Source: CAD feature listing. Evaluate the final solid. Frame: model axes, mm. A direction names the side the tool comes from. Round coordinates to 2 decimals unless told otherwise and drop trailing zeros. Loops run counter-clockwise (first coordinate to the right, second up) from the corner with the lowest first, then second, coordinate; pieces in that order, holes last. Notation, with made-up numbers: (-16.5, 30) - (1.5, 30) arc R16 cw to (1.5, 39) - close; hole circle Ø10 at (-27.75, 7.5). An arc over 180 degrees is marked (long way). Use CSV: the item, a comma, the result in double quotes. Start each with the question number.
from build123d import *

# Parameters (mm, degrees)
F0_R     = 6.35
F0_R_2   = 4.7625
F1_DEPTH = 6.35
F2_R     = 32.0379747342
F3_ANGLE = 180


with BuildPart() as f1:
    # F0 (on Front) → F1 (new body)
    with BuildSketch(Plane.XZ):
        with BuildLine():
            add(Edge.make_bspline(
                [(-44.9317906939, -75.2959670142), (-42.504350489, -76.9309330496), (-40.0815580843, -78.574281615), (-37.0058182453, -78.848974732)],
                knots=[0, 0, 0, 0, 0.304878312, 0.304878312, 0.304878312, 0.304878312], degree=3))
            Line((-37.0058182453, -78.848974732), (-35.1899303496, -78.848974732))
            Line((-35.1899303496, -78.848974732), (138.0456507325, -78.848974732))
            ThreePointArc((138.0456507325, -78.848974732), (107.5329699783, -68.6644436224), (89.25483042, -42.1944988733))
            ThreePointArc((89.25483042, -42.1944988733), (72.9581507325, -28.048974732), (89.25483042, -13.9034505906))
            ThreePointArc((89.25483042, -13.9034505906), (107.5329699783, 12.5664941585), (138.0456507325, 22.751025268))
            Line((138.0456507325, 22.751025268), (-29.5108688384, 22.751025268))
            ThreePointArc((-29.5108688384, 22.751025268), (-23.7287326375, -9.9063657522), (-37.9096431739, -39.8870272468))
            ThreePointArc((-37.9096431739, -39.8870272468), (-36.8982172715, -41.4219866867), (-36.5434579184, -43.2256575657))
            ThreePointArc((-36.5434579184, -43.2256575657), (-39.6962005674, -47.7078542952), (-44.9802400795, -46.2556834486))
            ThreePointArc((-44.9802400795, -46.2556834486), (-45.2388732076, -46.4494635579), (-45.4986485664, -46.6417097247))
            ThreePointArc((-45.4986485664, -46.6417097247), (-44.8982077868, -47.9076096174), (-44.6921152233, -49.2934514277))
            ThreePointArc((-44.6921152233, -49.2934514277), (-48.2687720926, -53.9059542537), (-53.62657499, -51.5904403165))
            ThreePointArc((-53.62657499, -51.5904403165), (-53.9605685551, -51.7543648971), (-54.2956711641, -51.9160102225))
            ThreePointArc((-54.2956711641, -51.9160102225), (-54.0112987886, -52.8294235617), (-53.9152156835, -53.781242669))
            ThreePointArc((-53.9152156835, -53.781242669), (-57.9302793656, -58.484724911), (-63.2056073689, -55.2575905738))
            ThreePointArc((-63.2056073689, -55.2575905738), (-63.9341966135, -55.4550487206), (-64.6654456429, -55.6424169789))
            ThreePointArc((-64.6654456429, -55.6424169789), (-64.5940899046, -56.1138214868), (-64.5702249334, -56.589998255))
            ThreePointArc((-64.5702249334, -56.589998255), (-69.063627601, -61.3448897233), (-74.0648151174, -57.1273331041))
            ThreePointArc((-74.0648151174, -57.1273331041), (-74.3067807591, -57.1436245398), (-74.5488163621, -57.1588412904))
            ThreePointArc((-74.5488163621, -57.1588412904), (-74.5483033729, -57.1991961718), (-74.5481323724, -57.2395539515))
            ThreePointArc((-74.5481323724, -57.2395539515), (-79.4779726733, -61.9991131195), (-84.0613726764, -56.9050800143))
            ThreePointArc((-84.0613726764, -56.9050800143), (-84.4367274692, -56.8608221199), (-84.811766966, -56.8139674761))
            ThreePointArc((-84.811766966, -56.8139674761), (-90.5205103625, -60.6546823767), (-94.1086444598, -54.7838957332))
            ThreePointArc((-94.1086444598, -54.7838957332), (-94.5178427862, -54.6545521612), (-94.926012036, -54.5219969142))
            ThreePointArc((-94.926012036, -54.5219969142), (-96.9364048452, -56.9248041814), (-100.0044999501, -57.5588029495))
            ThreePointArc((-100.0044999501, -57.5588029495), (-102.555846588, -60.8409888487), (-105.3670203015, -63.9035721205))
            add(Edge.make_bspline(
                [(-105.3670203015, -63.9035721205), (-93.0623740032, -63.7395817927), (-65.1691332268, -63.6755764129), (-51.7450297958, -70.7164798851), (-44.9317906939, -75.2959670142)],
                knots=[0.5750167778, 0.5750167778, 0.5750167778, 0.5750167778, 0.7300492168, 0.9453128196, 0.9453128196, 0.9453128196, 0.9453128196], degree=3))
        make_face()
        with BuildLine():
            Line((-35.1899303496, -78.848974732), (-37.0058182453, -78.848974732))
            add(Edge.make_bspline(
                [(-37.0058182453, -78.848974732), (-36.4252596683, -78.9008241905), (-35.8214378024, -78.9039110297), (-35.1899303496, -78.848974732)],
                knots=[0.304878312, 0.304878312, 0.304878312, 0.304878312, 0.3624253505, 0.3624253505, 0.3624253505, 0.3624253505], degree=3))
        make_face()
        with BuildLine():
            ThreePointArc((89.25483042, -42.1944988733), (107.5329699783, -68.6644436224), (138.0456507325, -78.848974732))
            ThreePointArc((138.0456507325, -78.848974732), (173.9666752168, -63.9699992163), (188.8456507325, -28.048974732))
            ThreePointArc((188.8456507325, -28.048974732), (173.9666752168, 7.8720497523), (138.0456507325, 22.751025268))
            ThreePointArc((138.0456507325, 22.751025268), (107.5329699783, 12.5664941585), (89.25483042, -13.9034505906))
            ThreePointArc((89.25483042, -13.9034505906), (98.0354331918, -18.6834394706), (101.5331507325, -28.048974732))
            ThreePointArc((101.5331507325, -28.048974732), (98.0354331918, -37.4145099934), (89.25483042, -42.1944988733))
        make_face()
        with BuildLine():
            add(Edge.make_bspline(
                [(-192.1543492675, -28.048974732), (-187.686217537, -40.4827740106), (-178.5952669037, -65.7808319564), (-128.5743222399, -64.2128677281), (-105.3670203015, -63.9035721205)],
                knots=[0, 0, 0, 0, 0.2826162867, 0.5750167778, 0.5750167778, 0.5750167778, 0.5750167778], degree=3))
            ThreePointArc((-105.3670203015, -63.9035721205), (-102.555846588, -60.8409888487), (-100.0044999501, -57.5588029495))
            ThreePointArc((-100.0044999501, -57.5588029495), (-103.5707491501, -55.1009846293), (-103.6714716912, -50.7709893382))
            ThreePointArc((-103.6714716912, -50.7709893382), (-99.8239881538, -48.0955305832), (-95.5471956554, -50.0113215546))
            ThreePointArc((-95.5471956554, -50.0113215546), (-93.2496774257, -44.3762692721), (-91.6424653425, -38.5069189195))
            ThreePointArc((-91.6424653425, -38.5069189195), (-92.322764275, -38.2378672888), (-92.9978166414, -37.9559103416))
            ThreePointArc((-92.9978166414, -37.9559103416), (-99.7102448029, -27.0812609993), (-91.7522812468, -17.0819857164))
            ThreePointArc((-91.7522812468, -17.0819857164), (-104.2898917661, 6.6910020977), (-127.2022100568, 20.7399272413))
            ThreePointArc((-127.2022100568, 20.7399272413), (-134.2071897004, 22.2457378144), (-141.3543492675, 22.751025268))
            ThreePointArc((-141.3543492675, 22.751025268), (-177.2753737518, 7.8720497523), (-192.1543492675, -28.048974732))
        make_face()
        with Locations((-141.3543492675, -28.048974732)):
            Circle(F0_R, mode=Mode.SUBTRACT)
        with BuildLine():
            ThreePointArc((-94.6181004106, -52.8373460118), (-94.6957106902, -53.6936254977), (-94.926012036, -54.5219969142))
            ThreePointArc((-94.926012036, -54.5219969142), (-94.5178427862, -54.6545521612), (-94.1086444598, -54.7838957332))
            ThreePointArc((-94.1086444598, -54.7838957332), (-88.8904205988, -51.2790749892), (-84.7420081356, -56.0018181271))
            ThreePointArc((-84.7420081356, -56.0018181271), (-84.7594798917, -56.4093880167), (-84.811766966, -56.8139674761))
            ThreePointArc((-84.811766966, -56.8139674761), (-84.4367274692, -56.8608221199), (-84.0613726764, -56.9050800143))
            ThreePointArc((-84.0613726764, -56.9050800143), (-79.1836309389, -52.4787476242), (-74.5488163621, -57.1588412904))
            ThreePointArc((-74.5488163621, -57.1588412904), (-74.3067807591, -57.1436245398), (-74.0648151174, -57.1273331041))
            ThreePointArc((-74.0648151174, -57.1273331041), (-70.0758898462, -51.8858392268), (-64.6654456429, -55.6424169789))
            ThreePointArc((-64.6654456429, -55.6424169789), (-63.9341966135, -55.4550487206), (-63.2056073689, -55.2575905738))
            ThreePointArc((-63.2056073689, -55.2575905738), (-60.3500965193, -49.3220332559), (-54.2956711641, -51.9160102225))
            ThreePointArc((-54.2956711641, -51.9160102225), (-53.9605685551, -51.7543648971), (-53.62657499, -51.5904403165))
            ThreePointArc((-53.62657499, -51.5904403165), (-51.9313362155, -45.2256191577), (-45.4986485664, -46.6417097247))
            ThreePointArc((-45.4986485664, -46.6417097247), (-45.2388732076, -46.4494635579), (-44.9802400795, -46.2556834486))
            ThreePointArc((-44.9802400795, -46.2556834486), (-44.493317629, -39.6869933651), (-37.9096431739, -39.8870272468))
            ThreePointArc((-37.9096431739, -39.8870272468), (-23.7287326375, -9.9063657522), (-29.5108688384, 22.751025268))
            Line((-29.5108688384, 22.751025268), (-126.1978296966, 22.751025268))
            ThreePointArc((-126.1978296966, 22.751025268), (-126.7103690202, 21.7506448125), (-127.2022100568, 20.7399272413))
            ThreePointArc((-127.2022100568, 20.7399272413), (-104.2898917661, 6.6910020977), (-91.7522812468, -17.0819857164))
            ThreePointArc((-91.7522812468, -17.0819857164), (-87.9555754664, -16.6503904081), (-84.2371330367, -17.5304104022))
            ThreePointArc((-84.2371330367, -17.5304104022), (-75.2103646617, -18.6241555339), (-67.0173262512, -14.6804330141))
            ThreePointArc((-67.0173262512, -14.6804330141), (-55.0611893817, -12.7851430462), (-48.4676535929, -22.9373161489))
            ThreePointArc((-48.4676535929, -22.9373161489), (-49.4279804902, -27.4562803601), (-52.1429809347, -31.1941992836))
            ThreePointArc((-52.1429809347, -31.1941992836), (-70.8607841381, -40.4245535235), (-91.6424653425, -38.5069189195))
            ThreePointArc((-91.6424653425, -38.5069189195), (-93.2496774257, -44.3762692721), (-95.5471956554, -50.0113215546))
            ThreePointArc((-95.5471956554, -50.0113215546), (-94.8563327131, -51.3499294422), (-94.6181004106, -52.8373460118))
        make_face()
        with Locations((-77.8543492675, -2.648974732)):
            Circle(F0_R_2, mode=Mode.SUBTRACT)
        with BuildLine():
            Line((-126.1978296966, 22.751025268), (-141.3543492675, 22.751025268))
            ThreePointArc((-141.3543492675, 22.751025268), (-134.2071897004, 22.2457378144), (-127.2022100568, 20.7399272413))
            ThreePointArc((-127.2022100568, 20.7399272413), (-126.7103690202, 21.7506448125), (-126.1978296966, 22.751025268))
        make_face()
    extrude(amount=F1_DEPTH)

    # F2
    f2_edges = [f1.edges().sort_by_distance(p)[0] for p in [
        (-192.154349, -3.175, -28.048975),
    ]]
    fillet(f2_edges, radius=F2_R)


with BuildPart() as f1_1:
    # F3: moved
    add(f1.part.rotate(Axis((-1.6543492675, -6.35, 22.751025268), (1, 0, 0)), F3_ANGLE))


solid = f1_1.part
1. Reachability of faces 1 (the flat face through (-4, -12.7, 73)), 2 (the cylindrical face through (-75.338, -9.569, 64.147)) from +Z, -Z, +X, -X, +Y, -Y: full face, straight path, thin tool, end or side. Return the list, or none.
2. Mould query, pull axis Z, two halves, no side actions, for faces 3 (the flat face through (0, -10, 22.751)), 4 (the flat face through (50, -10, 124.351)), 5 (the flat face through (-4, -6.35, 73)), 6 (the cylindrical face through (-82.612, -9.569, 47.942)). Classes: +Z half, -Z half, draft (parallel to the pull), parting line (faces both ways), or undercut.
3. Section query B-B on y = -9.25. Give the number of separate pieces and of enclosed holes in the cut face, and give its area (3 significant figures).
4. Section query C-C on x = 153. Return the cut outline in (y, z).
5. Contact query for flat-ended pins moving along their axis: P1, Ø1.9, axis at x = 10.5, y = -8.5, coming from the +Z side; P2, Ø2, axis at y = -7.5, z = 42.5, coming from the +X side; P3, Ø2, axis at x = -139.5, y = -9, coming from the +Z side. Output: stop coordinate, or through.
6. Section query A-A on x = 85. Return the cut outline in (y, z).
7. Line query: line 1 along X through (y, z) = (-12, 96); line 2 along Z through (x, y) = (-100, -11.5); line 3 along X through (y, z) = (-6.5, 61). Output: solid intervals per line, ascending.
Values:
1,face 1,"+Z, -Z, +X, -X, -Y"
1,face 2,"+Y, -Y"
2,face 3,"-Z half"
2,face 4,"+Z half"
2,face 5,"draft"
2,face 6,"undercut"
3,separate pieces,"1"
3,enclosed holes,"11"
3,area,"32,100 mm^2"
4,outline,"(-12.7, 25) - (-6.35, 25) - (-6.35, 122.1) - (-12.7, 122.1) - close"
5,P1,"stops at z = 124.35"
5,P2,"stops at x = 179"
5,P3,"stops at z = 109.38"
6,outline,"(-12.7, 22.75) - (-6.35, 22.75) - (-6.35, 59.44) - (-12.7, 59.44) - close; (-12.7, 87.66) - (-6.35, 87.66) - (-6.35, 124.35) - (-12.7, 124.35) - close"
7,line 1,"x = -180.74 to -103.53, -95.23 to -62.13, -55.23 to -54.06, -44.85 to 183.62"
7,line 2,"z = 22.75 to 93.62, 103.06 to 109.35"
7,line 3,"x = -190.58 to -68, -51.33 to 80.42, 94.07 to 187.27"
